Could you check a few things on this model? Use its own coordinates, in mm. A direction names the side the tool comes from. Round coordinates to 2 decimals unless told otherwise and drop trailing zeros. Loops run counter-clockwise (first coordinate to the right, second up) from the corner with the lowest first, then second, coordinate; pieces in that order, holes last. Notation, with made-up numbers: (18, -2) -> (76, -2) arc R25 ccw to (76, 27) -> close; hole circle Ø4 at (-38.75, 40.25). An arc over 180 degrees is marked (long way). One line per item, written item: value.
```python
from build123d import *

# Parameters (mm, degrees)
SKETCH1_R           = 1.75
SKETCH1_R_2         = 11.5
BOSS_EXTRUDE1_DEPTH = 4
CHAMFER1_SIZE       = 10
CHAMFER2_SIZE       = 10
CUT_EXTRUDE1_DEPTH  = 10
CUT_EXTRUDE2_DEPTH  = 10
FILLET1_R           = 15


with BuildPart() as part:
    # Sketch1 → Boss-Extrude1 (new body)
    with BuildSketch(Plane.XY):
        Polygon((-39.680258263, -5.004819249), (0.319741737, -5.004819249), (0.319741737, 4.995180751), (498.319741737, 4.995180751), (498.319741737, -5.004819249), (540.319741737, -5.004819249), (540.319741737, -420.004819249), (498.319741737, -420.004819249), (498.319741737, -460.004819249), (2.319741737, -460.004819249), (2.319741737, -420.004819249), (-39.680258263, -420.004819249), align=None)
        with Locations((457.319741737, -35.448212978)):
            Circle(SKETCH1_R, mode=Mode.SUBTRACT)
        with Locations((457.319741737, -66.448212978)):
            Circle(SKETCH1_R, mode=Mode.SUBTRACT)
        with Locations((488.319741737, -66.448212978)):
            Circle(SKETCH1_R, mode=Mode.SUBTRACT)
        with Locations((488.319741737, -35.448212978)):
            Circle(SKETCH1_R, mode=Mode.SUBTRACT)
        with Locations((472.819741737, -50.948212978)):
            Circle(SKETCH1_R_2, mode=Mode.SUBTRACT)
    extrude(amount=BOSS_EXTRUDE1_DEPTH)

    # Chamfer1
    chamfer1_edges = [part.edges().sort_by_distance(p)[0] for p in [
        (498.319741737, 4.995180751, 2),
        (0.319741737, 4.995180751, 2),
    ]]
    chamfer(chamfer1_edges, length=CHAMFER1_SIZE - 0.0001)  # a hair under: the kernel refuses the full size

    # Chamfer2
    chamfer2_edges = [part.edges().sort_by_distance(p)[0] for p in [
        (540.319741737, -5.004819249, 2),
        (540.319741737, -420.004819249, 2),
        (498.319741737, -460.004819249, 2),
        (2.319741737, -460.004819249, 2),
        (-39.680258263, -420.004819249, 2),
        (-39.680258263, -5.004819249, 2),
    ]]
    chamfer(chamfer2_edges, length=CHAMFER2_SIZE)

    # Sketch2 → Cut-Extrude1 (cut)
    with BuildSketch(Plane.XY.offset(4)):
        with BuildLine():
            Line((-20.680258263, -110.333406017), (519.319741737, -110.333406017))
            ThreePointArc((519.319741737, -110.333406017), (534.319741737, -125.333406017), (519.319741737, -140.333406017))
            Line((519.319741737, -140.333406017), (-20.680258263, -140.333406017))
            ThreePointArc((-20.680258263, -140.333406017), (-35.680258263, -125.333406017), (-20.680258263, -110.333406017))
        make_face()
    extrude(amount=-CUT_EXTRUDE1_DEPTH, mode=Mode.SUBTRACT)

    # Sketch3 → Cut-Extrude2 (cut)
    with BuildSketch(Plane(origin=(0, 0, 0), x_dir=(-1, 0, 0), z_dir=(0, 0, -1))):
        with BuildLine():
            Line((-273.763542149, -140.333406017), (-273.763542149, -340.333406017))
            ThreePointArc((-273.763542149, -340.333406017), (-258.763542149, -355.333406017), (-243.763542149, -340.333406017))
            Line((-243.763542149, -340.333406017), (-243.763542149, -140.333406017))
            Line((-243.763542149, -140.333406017), (-273.763542149, -140.333406017))
        make_face()
    extrude(amount=-CUT_EXTRUDE2_DEPTH, mode=Mode.SUBTRACT)

    # Fillet1
    fillet1_edges = [part.edges().sort_by_distance(p)[0] for p in [
        (273.763542149, -140.333406017, 2),
        (243.763542149, -140.333406017, 2),
    ]]
    fillet(fillet1_edges, radius=FILLET1_R)


solid = part.part
```
Item 1: If we section it at C-C on y = -428: List the corners of the cut face in (x, z) for me, plus the area to 3 significant figures.
Output:
outline: (2.32, 0) -> (498.32, 0) -> (498.32, 4) -> (2.32, 4) -> close
area: 1,980 mm²
Item 2: If we section it at B-B on x = 329.5: List the corners of the cut face in (y, z) for me.
Output:
outline: (-460, 0) -> (-140.33, 0) -> (-140.33, 4) -> (-460, 4) -> close; (-110.33, 0) -> (5, 0) -> (5, 4) -> (-110.33, 4) -> close
Item 3: If we section it at A-A on y = -174: List the corners of the cut face in (x, z) for me, plus the area to 3 significant figures.
Output:
outline: (-39.68, 0) -> (243.76, 0) -> (243.76, 4) -> (-39.68, 4) -> close; (273.76, 0) -> (540.32, 0) -> (540.32, 4) -> (273.76, 4) -> close
area: 2,200 mm²
Item 4: Will this pin go through, and if not, where does the flat tip stop? pin 1 Ø2 at (y, z) = (-430, 2.5) entering from +X.
Output:
pin 1: stops at x = 498.32
Item 5: For faces 1 (the face through (319, -224, 4)), 2 (the face through (278.274, -144.611, 2.028)), which set-ups out of +Z, -Z, +X, -X, +Y, -Y let a thin tool reach every point of the face, with its end or its side?
Output:
face 1: +Z, +X, -X, +Y, -Y
face 2: +Z, -Z
Item 6: If we mould it in two halves opening along X, with no side actions, what happens to faces 3 (the face through (319, -224, 0)), 4 (the face through (239.486, -144.844, 2.028)), 5 (the face through (534.316, -125.004, 2.028))? For each: released by +X, released by -X, zero draft, split by the parting line, or undercut.
Output:
face 3: zero draft
face 4: undercut
face 5: undercut
Item 7: If we section it at D-D on z = 1.7: Count the separate pieces of the cut face and the enclosed holes in it, plus the area to 3 significant figures.
Output:
separate pieces: 1
enclosed holes: 6
area: 241,000 mm²
Item 8: I need wall thicknesses on line 1 (Y direction, x = 185, z = 3.8); line 2 (Y direction, x = 464.5, z = 3.75); line 3 (X direction, y = -336.5, z = 1.75). Which ranges of each line are inside material? Lowest first, please. Write a range as from..to.
Output:
line 1: y = -460..-140.33, -110.33..5
line 2: y = -460..-140.33, -110.33..-58.89, -43.01..5
line 3: x = -39.68..243.76, 273.76..540.32
